```python
from build123d import *

# Parameters (mm, degrees)
SKETCH2_W           = 13.5
SKETCH2_H           = 3.5
SKETCH2_R           = 1.75
BOSS_EXTRUDE2_DEPTH = 12
BOSS_EXTRUDE3_START = 12
SKETCH2_4_W         = 6
SKETCH2_4_H         = 10
BOSS_EXTRUDE3_DEPTH = 5
CUT_EXTRUDE1_START  = 12
SKETCH2_6_W         = 13.5
SKETCH2_6_H         = 1.5
CUT_EXTRUDE1_DEPTH  = 9.3
CUT_EXTRUDE2_START  = 12
CUT_EXTRUDE2_DEPTH  = 4.5
CUT_EXTRUDE3_START  = 3.5
SKETCH2_8_R         = 3.5
SKETCH2_8_R_2       = 1.75
CUT_EXTRUDE3_DEPTH  = 8.5
FILLET1_R           = 3
CHAMFER1_SIZE       = 0.5
CUT_EXTRUDE4_DEPTH  = 1.5


with BuildPart() as part:
    # Sketch2 → Boss-Extrude2 (new body)
    with BuildSketch(Plane(origin=(0, 0, 0), x_dir=(1, 0, 0), z_dir=(0, 1, 0))):
        with BuildLine():
            Line((-18, -12.5), (18, -12.5))
            ThreePointArc((18, -12.5), (21.5, -16), (25, -12.5))
            Line((25, -12.5), (25, 12.5))
            ThreePointArc((25, 12.5), (21.5, 16), (18, 12.5))
            Line((18, 12.5), (-18, 12.5))
            ThreePointArc((-18, 12.5), (-21.5, 16), (-25, 12.5))
            Line((-25, 12.5), (-25, -12.5))
            ThreePointArc((-25, -12.5), (-21.5, -16), (-18, -12.5))
        make_face()
        with Locations((17, 0)):
            Rectangle(SKETCH2_W, SKETCH2_H, mode=Mode.SUBTRACT)
        with Locations(Location((-20, 0, 0), (0, 0, 270))):
            Circle(SKETCH2_R, mode=Mode.SUBTRACT)
        with Locations(Location((5, 0, 0), (0, 0, 270))):
            Circle(SKETCH2_R, mode=Mode.SUBTRACT)
    extrude(amount=BOSS_EXTRUDE2_DEPTH)

    # Sketch2<4> → Boss-Extrude3 (add)
    with BuildSketch(Plane(origin=(0, 0, 0), x_dir=(1, 0, 0), z_dir=(0, 1, 0)).offset(BOSS_EXTRUDE3_START)):
        with Locations((28, 0)):
            Rectangle(SKETCH2_4_W, SKETCH2_4_H)
    extrude(amount=-BOSS_EXTRUDE3_DEPTH)

    # Sketch2<6> → Cut-Extrude1 (cut)
    with BuildSketch(Plane(origin=(0, 0, 0), x_dir=(1, 0, 0), z_dir=(0, 1, 0)).offset(CUT_EXTRUDE1_START)):
        with Locations((17, -2.5)):
            Rectangle(SKETCH2_6_W, SKETCH2_6_H)
        with Locations((17, 2.5)):
            Rectangle(SKETCH2_6_W, SKETCH2_6_H)
    extrude(amount=-CUT_EXTRUDE1_DEPTH, mode=Mode.SUBTRACT)

    # Sketch2<7> → Cut-Extrude2 (cut)
    with BuildSketch(Plane(origin=(0, 0, 0), x_dir=(1, 0, 0), z_dir=(0, 1, 0)).offset(CUT_EXTRUDE2_START)):
        with BuildLine():
            ThreePointArc((23.65, 12.5), (21.5, 14.65), (19.35, 12.5))
            Line((19.35, 12.5), (23.65, 12.5))
        make_face()
        with BuildLine():
            Line((23.65, 12.5), (19.35, 12.5))
            ThreePointArc((19.35, 12.5), (21.5, 10.35), (23.65, 12.5))
        make_face()
        with BuildLine():
            ThreePointArc((23.65, -12.5), (21.5, -10.35), (19.35, -12.5))
            Line((19.35, -12.5), (23.65, -12.5))
        make_face()
        with BuildLine():
            Line((23.65, -12.5), (19.35, -12.5))
            ThreePointArc((19.35, -12.5), (21.5, -14.65), (23.65, -12.5))
        make_face()
        with BuildLine():
            ThreePointArc((-19.35, 12.5), (-21.5, 14.65), (-23.65, 12.5))
            Line((-23.65, 12.5), (-19.35, 12.5))
        make_face()
        with BuildLine():
            Line((-19.35, 12.5), (-23.65, 12.5))
            ThreePointArc((-23.65, 12.5), (-21.5, 10.35), (-19.35, 12.5))
        make_face()
        with BuildLine():
            ThreePointArc((-23.65, -12.5), (-21.5, -14.65), (-19.35, -12.5))
            Line((-19.35, -12.5), (-23.65, -12.5))
        make_face()
        with BuildLine():
            Line((-23.65, -12.5), (-19.35, -12.5))
            ThreePointArc((-19.35, -12.5), (-21.5, -10.35), (-23.65, -12.5))
        make_face()
    extrude(amount=-CUT_EXTRUDE2_DEPTH, mode=Mode.SUBTRACT)

    # Sketch2<8> → Cut-Extrude3 (cut)
    # profile 1 of 2: a face of its own
    with BuildSketch(Plane(origin=(0, 0, 0), x_dir=(1, 0, 0), z_dir=(0, 1, 0)).offset(CUT_EXTRUDE3_START)):
        with Locations(Location((-20, 0, 0), (0, 0, 270))):
            Circle(SKETCH2_8_R)
        with Locations(Location((-20, 0, 0), (0, 0, 270))):
            Circle(SKETCH2_8_R_2, mode=Mode.SUBTRACT)
    # profile 2 of 2: a face of its own
    with BuildSketch(Plane(origin=(0, 0, 0), x_dir=(1, 0, 0), z_dir=(0, 1, 0)).offset(CUT_EXTRUDE3_START)):
        with Locations(Location((5, 0, 0), (0, 0, 270))):
            Circle(SKETCH2_8_R)
        with Locations(Location((5, 0, 0), (0, 0, 270))):
            Circle(SKETCH2_8_R_2, mode=Mode.SUBTRACT)
    extrude(amount=CUT_EXTRUDE3_DEPTH, mode=Mode.SUBTRACT)

    # Fillet1
    fillet1_edges = [part.edges().sort_by_distance(p)[0] for p in [
        (25, 9.5, -5),
        (25, 9.5, 5),
    ]]
    fillet(fillet1_edges, radius=FILLET1_R)

    # Chamfer1
    chamfer1_edges = [part.edges().sort_by_distance(p)[0] for p in [
        (19.35, 12, 12.5),
        (-23.65, 12, -12.5),
        (-19.35, 12, 12.5),
        (19.35, 12, -12.5),
    ]]
    chamfer(chamfer1_edges, length=CHAMFER1_SIZE)

    # Sketch3 → Cut-Extrude4 (cut)
    with BuildSketch(Plane.XZ):
        Polygon((10.25, 1.75), (10.25, 12.5), (14.25, 12.5), (23.75, 1.75), align=None)
    extrude(amount=-CUT_EXTRUDE4_DEPTH, mode=Mode.SUBTRACT)


solid = part.part
```
Check sheet for the modelled part. Datum: model origin and axes. Units: mm. A direction names the side the tool comes from. Round coordinates to 2 decimals unless told otherwise and drop trailing zeros. Order: outer loops, then holes, each group sorted by start corner. A loop starts at its lowest first (then second) coordinate and runs counter-clockwise, first axis right, second up. Notation, with made-up numbers: M 41.25,32 L 59.25,32 A36 cw 59.25,69 Z; hole C 79,67 d10. An arc over 180 degrees is marked long. Answer in a Markdown table with one row per item.
(1) Gauge pin test, flat ends, axial feed: pin 1 (6 mm diameter, centred on x = -6, y = 9, fed in from +Z); pin 2 (3.5 mm diameter, centred on x = 21.5, z = 12.5, fed in from +Y); pin 3 (6 mm diameter, centred on x = 16, y = 8.5, fed in from +Z). Record the tip position at first contact, or that the pin passes through.
Findings:
| item | result |
|---|---|
| pin 1 | stops at z = 12.5 |
| pin 2 | stops at y = 7.5 |
| pin 3 | stops at z = 14.95 |
(2) Section check B-B on x = 5. Record the boundary of the cut face in (y, z).
Findings:
| item | result |
|---|---|
| outline | M 0,-12.5 L 12,-12.5 L 12,-3.5 L 3.5,-3.5 L 3.5,-1.75 L 0,-1.75 Z; M 0,1.75 L 3.5,1.75 L 3.5,3.5 L 12,3.5 L 12,12.5 L 0,12.5 Z |
(3) Draft check along X on faces 1 (the flat face through (29, 10, -5)), 2 (the flat face through (4, 3.5, -2)), 3 (the flat face through (-25, 6, 0)). Enter one of: +X half, -X half, draft (parallel to the pull), parting line (faces both ways), or undercut.
Findings:
| item | result |
|---|---|
| face 1 | draft |
| face 2 | undercut |
| face 3 | -X half |
(4) Set-up check for faces 4 (the cylindrical face through (21.4, 5.9, 16)), 5 (the flat face through (17, 1, -1.75)), 6 (the flat face through (16, 1.5, 6)), 7 (the flat face through (0, 6, -12.5)), 8 (the flat face through (-18, 3.5, 1)): record each of +Z, -Z, +X, -X, +Y, -Y from which the full face is reachable in a straight line by a thin tool's end or side.
Findings:
| item | result |
|---|---|
| face 4 | +Z, +Y, -Y |
| face 5 | +Y, -Y |
| face 6 | -Y |
| face 7 | -Z, +Y, -Y |
| face 8 | +Y |
(5) Material ranges on line 1 along X through (y, z) = (2.4, 0); line 2 along X through (y, z) = (7.75, 0); line 3 along Z through (x, y) = (21.5, 10.4), recorded low to high. Write a range as from..to.
Findings:
| item | result |
|---|---|
| line 1 | x = -25..-21.75, -18.25..3.25, 6.75..10.25, 23.75..25 |
| line 2 | x = -25..-23.5, -16.5..1.5, 8.5..10.25, 23.75..31 |
| line 3 | z = -16..-14.65, -10.35..-3.25, 3.25..10.35, 14.65..16 |
(6) Section check C-C on x = -2. Record the boundary of the cut face in (y, z).
Findings:
| item | result |
|---|---|
| outline | M 0,-12.5 L 12,-12.5 L 12,12.5 L 0,12.5 Z |
(7) Section check A-A on z = 0. Record the boundary of the cut face in (x, y), plus the area to 4 significant figures.
Findings:
| item | result |
|---|---|
| outline | M -25,0 L -21.75,0 L -21.75,3.5 L -23.5,3.5 L -23.5,12 L -25,12 Z; M -18.25,0 L 3.25,0 L 3.25,3.5 L 1.5,3.5 L 1.5,12 L -16.5,12 L -16.5,3.5 L -18.25,3.5 Z; M 6.75,0 L 10.25,0 L 10.25,12 L 8.5,12 L 8.5,3.5 L 6.75,3.5 Z; M 23.75,0 L 25,0 L 25,7 L 31,7 L 31,12 L 23.75,12 Z |
| area | 324.5 mm^2 |
